The drawing under review shows one solid part. Ordinate dimensions are in mm from its lowest x, y, z. Round coordinates to 2 decimals unless told otherwise and drop trailing zeros. Order: outer loops, then holes, each group sorted by start corner. A loop starts at its lowest first (then second) coordinate and runs counter-clockwise, first axis right, second up.
1) To check wall thickness, follow L1, parallel to Y at x = 174, z = 8.75; L2, parallel to Y at x = 36, z = 1.5. State the ranges of each line that lie inside material, in increasing order.
2) Mouldability with a two-part tool opening along X and no side actions: class the marked faces 1, 2 and 3 as pulls with the +X half, pulls with the -X half, needs draft (parallel to the pull), parting line crosses it, or undercut.
3) Clearance check with flat-ended pins moving along their axes: P1, Ø1, axis at x = 135, z = 12, coming from the -Y side; P2, Ø3, axis at y = 3, z = 10.5, coming from the -X side. State where each tip first meets the part, or that it passes through.
4) Consider section A-A (z = 2.25). Give the number of separate pieces and of enclosed holes in the cut face, then the cut area to 3 significant figures.
5) Consider section B-B (x = 170). Give the boundary of the cut face in (y, z).
6) Consider section C-C (x = 59.5). Give the boundary of the cut face in (y, z).
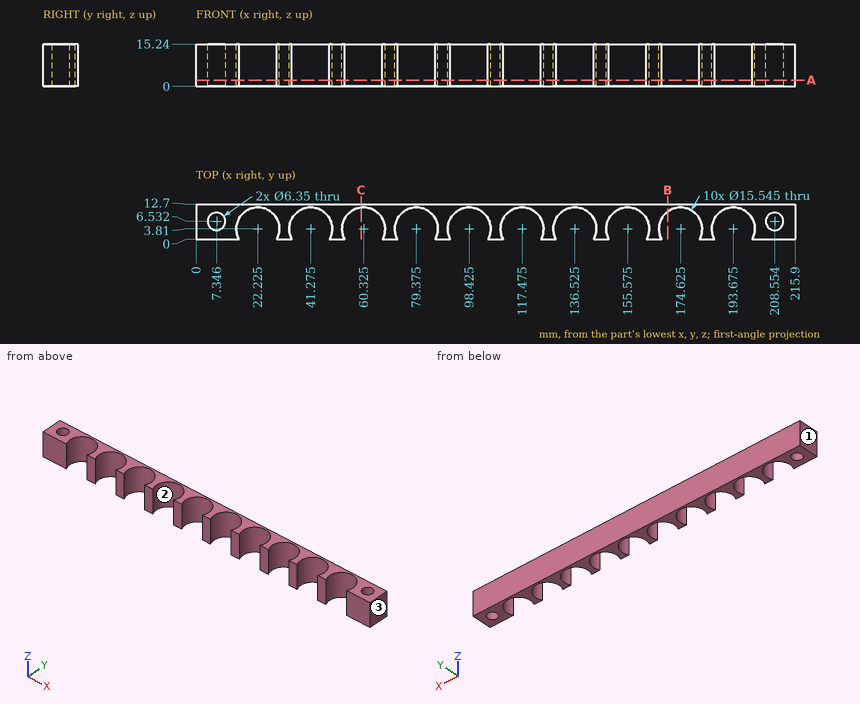
Answer below:
1. L1: y = 11.56 to 12.7
1. L2: y = 9.52 to 12.7
2. face 1: pulls with the -X half
2. face 2: undercut
2. face 3: pulls with the +X half
3. P1: stops at y = 11.31
3. P2: stops at x = 0
4. separate pieces: 1
4. enclosed holes: 2
4. area: 1,160 mm2
5. outline: (10.06, 0) - (12.7, 0) - (12.7, 15.24) - (10.06, 15.24) - close
6. outline: (11.54, 0) - (12.7, 0) - (12.7, 15.24) - (11.54, 15.24) - close
